Source: CAD feature listing. Evaluate the final solid. Frame: model axes, mm. A direction names the side the tool comes from. Coordinates: 2 decimals unless noted, no trailing zeros. Write each loop counter-clockwise with the first axis right and the second up, starting at its lowest first coordinate (ties: lowest second). Pieces come first, ordered by that corner, then holes. Notation, with made-up numbers: M 47,-24 L 82,-24 A23 cw 82,-13 Z; hole C 58,39.25 d8. An arc over 180 degrees is marked long. Answer as CSV lines item,"result". Start each with the question number.
1. Section D-D on x = -5.5. Return the cut outline in (y, z).
2. Section A-A on x = 5.25. Return the cut outline in (y, z), plus the area to 3 significant figures.
3. Section B-B on z = -2.54. Return the cut outline in (x, y).
4. Line query: probe 1 along Y at (x, z) = (-4.5, -2.54); probe 2 along Z at (x, y) = (4, -0.2); probe 3 along X at (y, z) = (0.95, 0). Output: solid intervals per line, ascending. Write a range as [from, to].
5. Contact query for flat-ended pins moving along their axis: pin 1 Ø1 at (y, z) = (0, 0) entering from -X; pin 2 Ø1.2 at (y, z) = (0, 0.5) entering from -X; pin 3 Ø0.8 at (x, z) = (2.5, -2.5) entering from +Y; pin 4 Ø0.8 at (x, z) = (0.5, 2.5) entering from +Y. Output: stop coordinate, or through.
6. Reachability of faces 4 (the face through (2, 0.724, 3)), 5 (the face through (0, 1.232, -3)), 6 (the face through (-4.252, 0.229, -1.813)) from +Z, -Z, +X, -X, +Y, -Y: full face, straight path, thin tool, end or side. Return the list, or none.
7. Section C-C on x = 2.25. Return the cut outline in (y, z), plus the area to 3 significant figures.
8. Mould query, pull axis Z, two halves, no side actions, for faces 1 (the face through (0, 0, 3.81)), 2 (the face through (0, 1.232, 3)), 3 (the face through (-4.252, 0.229, 3.267)). Classes: pulls with the +Z half, pulls with the -Z half, needs draft (parallel to the pull), parting line crosses it, or undercut.
```python
from build123d import *

# Parameters (mm, degrees)
SKETCH1_W           = 14.0208
SKETCH1_H           = 7.62
BOSS_EXTRUDE1_DEPTH = 1.3081
SKETCH2_W           = 0.762
SKETCH2_H           = 0.762
CUT_EXTRUDE1_DEPTH  = 6.35
CHAMFER1_SIZE       = 0.508
SKETCH3_W           = 1.778
SKETCH3_H           = 1.778
CUT_EXTRUDE2_DEPTH  = 0.254
SKETCH4_R           = 0.762
CUT_EXTRUDE3_DEPTH  = 5.08
SKETCH5_W           = 5.0038
SKETCH5_H           = 0.6604
CUT_EXTRUDE4_DEPTH  = 8.62
SKETCH6_W           = 1.524
SKETCH6_H           = 0.381
SKETCH6_H_2         = 0.762
SKETCH6_H_3         = 1.524
CUT_EXTRUDE5_DEPTH  = 0.254
SKETCH7_W           = 1.524
SKETCH7_H           = 0.254
BOSS_EXTRUDE2_DEPTH = 3.4798


with BuildPart() as part:
    # Sketch1 → Boss-Extrude1 (new body, symmetric)
    with BuildSketch(Plane(origin=(0, 0, 0), x_dir=(1, 0, 0), z_dir=(0, 1, 0))):
        Rectangle(SKETCH1_W, SKETCH1_H)
    extrude(amount=BOSS_EXTRUDE1_DEPTH, both=True)

    # Sketch2 → Cut-Extrude1 (cut)
    with BuildSketch(Plane(origin=(7.0104, 0, 0), x_dir=(0, 0, -1), z_dir=(1, 0, 0))):
        Rectangle(SKETCH2_W, SKETCH2_H)
        with Locations((-2.54, 0)):
            Rectangle(SKETCH2_W, SKETCH2_H)
        with Locations((2.54, 0)):
            Rectangle(SKETCH2_W, SKETCH2_H)
    extrude(amount=-CUT_EXTRUDE1_DEPTH, mode=Mode.SUBTRACT)

    # Chamfer1
    chamfer1_edges = [part.edges().sort_by_distance(p)[0] for p in [
        (7.0104, -0.381, 2.54),
        (7.0104, 0, 2.159),
        (7.0104, 0.381, 2.54),
        (7.0104, 0, 2.921),
        (7.0104, -0.381, 0),
        (7.0104, 0, -0.381),
        (7.0104, 0.381, 0),
        (7.0104, 0, 0.381),
        (7.0104, -0.381, -2.54),
        (7.0104, 0, -2.921),
        (7.0104, 0.381, -2.54),
        (7.0104, 0, -2.159),
    ]]
    chamfer(chamfer1_edges, length=CHAMFER1_SIZE)

    # Sketch3 → Cut-Extrude2 (cut)
    with BuildSketch(Plane.ZY.offset(7.0104)):
        with Locations((-2.54, 0)):
            Rectangle(SKETCH3_W, SKETCH3_H)
        Rectangle(SKETCH3_W, SKETCH3_H)
        with Locations((2.54, 0)):
            Rectangle(SKETCH3_W, SKETCH3_H)
    extrude(amount=-CUT_EXTRUDE2_DEPTH, mode=Mode.SUBTRACT)

    # Sketch4 → Cut-Extrude3 (cut)
    with BuildSketch(Plane.ZY.offset(6.7564)):
        with Locations((-2.54, 0)):
            Circle(SKETCH4_R)
        Circle(SKETCH4_R)
        with Locations((2.54, 0)):
            Circle(SKETCH4_R)
    extrude(amount=-CUT_EXTRUDE3_DEPTH, mode=Mode.SUBTRACT)

    # Sketch5 → Cut-Extrude4 (cut, through all)
    with BuildSketch(Plane.XY.offset(3.81)):
        with Locations((0.5715, 1.3081)):
            Rectangle(SKETCH5_W, SKETCH5_H)
    extrude(amount=-CUT_EXTRUDE4_DEPTH, mode=Mode.SUBTRACT)

    # Sketch6 → Cut-Extrude5 (cut)
    with BuildSketch(Plane(origin=(0, 0.9779, 0), x_dir=(1, 0, 0), z_dir=(0, 1, 0))):
        with Locations((2.3114, 3.1115)):
            Rectangle(SKETCH6_W, SKETCH6_H)
        with Locations((2.3114, 2.54)):
            Rectangle(SKETCH6_W, SKETCH6_H_2)
        with Locations((2.3114, 1.9685)):
            Rectangle(SKETCH6_W, SKETCH6_H)
        with Locations((2.3114, 0)):
            Rectangle(SKETCH6_W, SKETCH6_H_3)
        with Locations((2.3114, -2.54)):
            Rectangle(SKETCH6_W, SKETCH6_H_3)
    extrude(amount=-CUT_EXTRUDE5_DEPTH, mode=Mode.SUBTRACT)

    # Sketch7 → Boss-Extrude2 (add)
    with BuildSketch(Plane(origin=(-1.9304, 0, 0), x_dir=(0, 0, -1), z_dir=(1, 0, 0))):
        with Locations((2.54, 1.1049)):
            Rectangle(SKETCH7_W, SKETCH7_H)
        with Locations((0, 1.1049)):
            Rectangle(SKETCH7_W, SKETCH7_H)
        with Locations((-2.54, 1.1049)):
            Rectangle(SKETCH7_W, SKETCH7_H)
    extrude(amount=BOSS_EXTRUDE2_DEPTH)


solid = part.part
```
Values:
1,outline,"M -1.31,-3.81 L 1.31,-3.81 L 1.31,3.81 L -1.31,3.81 Z; hole C 0,-2.54 d1.52; hole C 0,0 d1.52; hole C 0,2.54 d1.52"
2,outline,"M -1.31,-3.81 L 1.31,-3.81 L 1.31,3.81 L -1.31,3.81 Z; hole M -0.38,-2.92 L 0.38,-2.92 L 0.38,-2.16 L -0.38,-2.16 Z; hole M -0.38,-0.38 L 0.38,-0.38 L 0.38,0.38 L -0.38,0.38 Z; hole M -0.38,2.16 L 0.38,2.16 L 0.38,2.92 L -0.38,2.92 Z"
2,area,"18.2 mm²"
3,outline,"M -7.01,-1.31 L 7.01,-1.31 L 7.01,-0.89 L 6.5,-0.38 L 0.66,-0.38 L 0.66,0.38 L 6.5,0.38 L 7.01,0.89 L 7.01,1.31 L 3.07,1.31 L 3.07,0.72 L 1.55,0.72 L 1.55,1.23 L -1.93,1.23 L -1.93,1.31 L -7.01,1.31 L -7.01,0.89 L -6.76,0.89 L -6.76,0.76 L -1.68,0.76 L -1.68,-0.76 L -6.76,-0.76 L -6.76,-0.89 L -7.01,-0.89 Z"
4,probe 1,"[-1.31, -0.76], [0.76, 1.31]"
4,probe 2,"[-3.81, -2.92], [-2.16, -0.38], [0.38, 2.16], [2.92, 3.81]"
4,probe 3,"[-7.01, 1.55], [3.07, 7.01]"
5,pin 1,"x = -1.68"
5,pin 2,"x = -7.01"
5,pin 3,"y = 0.72"
5,pin 4,"y = 1.23"
6,face 4,"+Y"
6,face 5,"+Z, -Z, +Y"
6,face 6,"-X"
7,outline,"M -1.31,-3.81 L 0.98,-3.81 L 0.98,-3.3 L 0.72,-3.3 L 0.72,-1.78 L 0.98,-1.78 L 0.98,-0.76 L 0.72,-0.76 L 0.72,0.76 L 0.98,0.76 L 0.98,1.78 L 0.72,1.78 L 0.72,3.3 L 0.98,3.3 L 0.98,3.81 L -1.31,3.81 Z; hole M -0.38,-2.92 L 0.38,-2.92 L 0.38,-2.16 L -0.38,-2.16 Z; hole M -0.38,-0.38 L 0.38,-0.38 L 0.38,0.38 L -0.38,0.38 Z; hole M -0.38,2.16 L 0.38,2.16 L 0.38,2.92 L -0.38,2.92 Z"
7,area,"14.5 mm²"
8,face 1,"pulls with the +Z half"
8,face 2,"needs draft"
8,face 3,"undercut"
